```python
from build123d import *

# Parameters (mm, degrees)
SKETCH_R        = 7.5
PAD_DEPTH       = 3.5
SKETCH001_R     = 5
PAD001_DEPTH    = 51
SKETCH002_R     = 2.075
POCKET_DEPTH    = 54.501
SKETCH003_R     = 3.6
POCKET001_DEPTH = 5


with BuildPart() as part:
    # Sketch → Pad (new body)
    with BuildSketch(Plane.XY):
        Circle(SKETCH_R)
    extrude(amount=PAD_DEPTH)

    # Sketch001 (on Face3 of Pad) → Pad001 (join)
    with BuildSketch(Plane.XY.offset(3.5)):
        Circle(SKETCH001_R)
    extrude(amount=PAD001_DEPTH)

    # Sketch002 (on Face2 of Pad001) → Pocket (cut, through all)
    with BuildSketch(Plane(origin=(0, 0, 0), x_dir=(1, 0, 0), z_dir=(0, 0, -1))):
        Circle(SKETCH002_R)
    extrude(amount=-POCKET_DEPTH, mode=Mode.SUBTRACT)

    # Sketch003 (on Face2 of Pocket) → Pocket001 (cut)
    with BuildSketch(Plane(origin=(0, 0, 0), x_dir=(1, 0, 0), z_dir=(0, 0, -1))):
        Circle(SKETCH003_R)
    extrude(amount=-POCKET001_DEPTH, mode=Mode.SUBTRACT)


solid = part.part
```
Source: CAD feature listing. Evaluate the final solid. Frame: model axes, mm. A direction names the side the tool comes from. Give positions to 0.01 mm unless a question says otherwise; leave off trailing zeros. Loops run counter-clockwise (first coordinate to the right, second up) from the corner with the lowest first, then second, coordinate; pieces in that order, holes last. Notation, with made-up numbers: M -4,25 L 23,25 A24 ccw 23,41 Z; hole C 56.5,46.5 d5. An arc over 180 degrees is marked long. Put each result on its own line as item: value.
Q1. Section B-B (y = 1.25). Return the cut outline in (x, z), and give its area (3 significant figures).
Response values:
outline: M -7.4,0 L -3.38,0 L -3.38,5 L -1.66,5 L -1.66,54.5 L -4.84,54.5 L -4.84,3.5 L -7.4,3.5 Z; M 1.66,5 L 3.38,5 L 3.38,0 L 7.4,0 L 7.4,3.5 L 4.84,3.5 L 4.84,54.5 L 1.66,54.5 Z
area: 348 mm²
Q2. Line query: probe 1 along Y at (x, z) = (0, 3.2); probe 2 along Z at (x, y) = (-5.5, 0.75); probe 3 along Z at (x, y) = (-0.25, 3.25). Output: solid intervals per line, ascending. Write a range as [from, to].
Response values:
probe 1: y = [-7.5, -3.6], [3.6, 7.5]
probe 2: z = [0, 3.5]
probe 3: z = [5, 54.5]
Q3. Pin query (flat end, axial travel): P1, Ø8, axis at x = -0.5, y = 0, coming from the -Z side; P2, Ø4, axis at x = -3.5, z = 32, coming from the +Y side; P3, Ø5, axis at x = 2, z = 40, coming from the -Y side; P4, Ø1, axis at x = -1.5, y = 2, coming from the -Z side. Return the tip coordinate at first contact, or that it passes through.
Response values:
P1: stops at z = 0
P2: stops at y = 4.77
P3: stops at y = -5
P4: stops at z = 5
Q4. Mould query, pull axis X, two halves, no side actions, for faces 4 (the flat face through (1, -2, 54.5)), 5 (the cylindrical face through (-1.08, -4.88, 28.64)), 6 (the cylindrical face through (-0.45, 2.026, 29.404)). Classes: released by +X, released by -X, zero draft, split by the parting line, or undercut.
Response values:
face 4: zero draft
face 5: split by the parting line
face 6: undercut
Q5. Section D-D (x = -4.25). Return the cut outline in (y, z), and give its area (3 significant figures).
Response values:
outline: M -6.18,0 L 6.18,0 L 6.18,3.5 L 2.63,3.5 L 2.63,54.5 L -2.63,54.5 L -2.63,3.5 L -6.18,3.5 Z
area: 312 mm²
Q6. Section C-C (z = 40). Return the cut outline in (x, y) (3 decimals), and give its area (3 significant figures).
Response values:
outline: C 0,0 d10; hole C 0,0 d4.15
area: 65.0 mm²
Q7. Section A-A (x = 0). Return the cut outline in (y, z) (3 decimals), and give its area (3 significant figures).
Response values:
outline: M -7.5,0 L -3.6,0 L -3.6,5 L -2.075,5 L -2.075,54.5 L -5,54.5 L -5,3.5 L -7.5,3.5 Z; M 2.075,5 L 3.6,5 L 3.6,0 L 7.5,0 L 7.5,3.5 L 5,3.5 L 5,54.5 L 2.075,54.5 Z
area: 321 mm²
Q8. Reachability of faces 1 (the cylindrical face through (3.434, -1.081, 2.465)), 2 (the flat face through (2, -5, 3.5)), 3 (the flat face through (1.6, 3.4, 0)) from +Z, -Z, +X, -X, +Y, -Y: full face, straight path, thin tool, end or side. Return the list, or none.
Response values:
face 1: -Z
face 2: +Z
face 3: -Z, +X, -X, +Y, -Y
